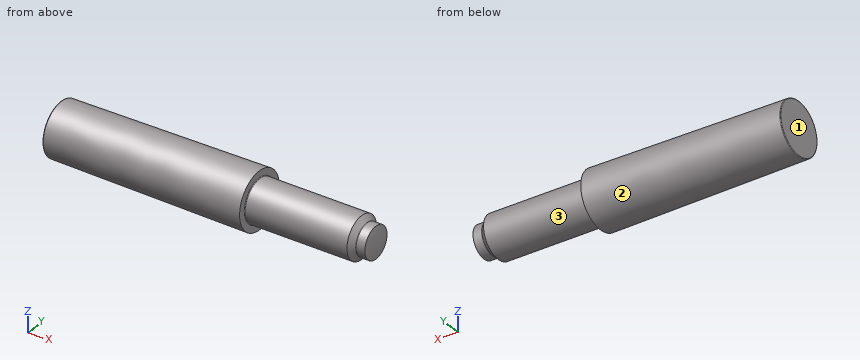
from build123d import *

# Parameters (mm, degrees)
FILLETS_R = 0.25


with BuildPart() as part:
    # BodySke → Body (revolve)
    with BuildSketch(Plane.XY, mode=Mode.PRIVATE) as body_sk:
        with BuildLine():
            Line((0, 0), (0, 10))
            Line((0, 10), (75, 10.749999999))
            Line((75, 10.749999999), (75, 8))
            Line((75, 8), (113.7, 8))
            Line((113.7, 8), (115.7, 6))
            Line((115.7, 6), (119.078784028, 6))
            ThreePointArc((119.078784028, 6), (119.768354516, 3.035153986), (120, 0))
            Line((120, 0), (0, 0))
        make_face()
    revolve(body_sk.sketch.rotate(Axis((-8.740321592, 0, 0), (1, 0, 0)), 90), axis=Axis((-8.740321592, 0, 0), (1, 0, 0)))

    # Fillets
    fillets_edges = [part.edges().sort_by_distance(p)[0] for p in [
        (0, 0, -10),
        (75, 0, -8),
        (115.7, 0, -6),
    ]]
    fillet(fillets_edges, radius=FILLETS_R)


solid = part.part
Model file for the job. Use its own axes, mm. Face numbers are marked on the shaded views. A direction names the side the tool comes from. Coordinates: 2 decimals unless noted, no trailing zeros. Write each loop counter-clockwise with the first axis right and the second up, starting at its lowest first coordinate (ties: lowest second). Pieces come first, ordered by that corner, then holes. Notation, with made-up numbers: (85.5, 69.25) -> (133.5, 69.25) arc R10 ccw to (133.5, 88.25) -> close; hole circle Ø3 at (76.5, 63). An arc over 180 degrees is marked (long way). One line per item, written item: value. Start each with the question number.
1) Probe probe 1 along Y at (x, z) = (60, 3.5); probe 2 along Z at (x, y) = (88, -0.5); probe 3 along Y at (x, z) = (83.5, 0). List the from-to ranges inside material, lowest first.
2) Flat gauge pins, fed straight in: pin 1 Ø8 at (x, z) = (36.5, -7.5) entering from -Y; pin 2 Ø4 at (x, y) = (30.5, -7) entering from +Z; pin 3 Ø8 at (x, y) = (37.5, 5.5) entering from -Z. Where does each tip first touch, or does it go through?
3) Which spindle directions (+Z, -Z, +X, -X, +Y, -Y) get a long thin tool onto all of the face, cutting with end or side? Do the marked faces 1, 2 and 3. Say none if no direction does.
4) Slice it at B-B on x = 72. Write the cut outline in (y, z), then the cut area to 3 significant figures.
5) Slice it at A-A on x = 87. Write the cut outline in (y, z), then the cut area to 3 significant figures.
Answers follow:
1. probe 1: -10.01 to 10.01
1. probe 2: -7.98 to 7.98
1. probe 3: -8 to 8
2. pin 1: y = -9.76
2. pin 2: z = 9.01
2. pin 3: z = -10.27
3. face 1: +Z, -Z, -X, +Y, -Y
3. face 2: -X
3. face 3: +X
4. outline: circle Ø21.44 at (0, 0)
4. area: 361 mm2
5. outline: circle Ø16 at (0, 0)
5. area: 201 mm2
